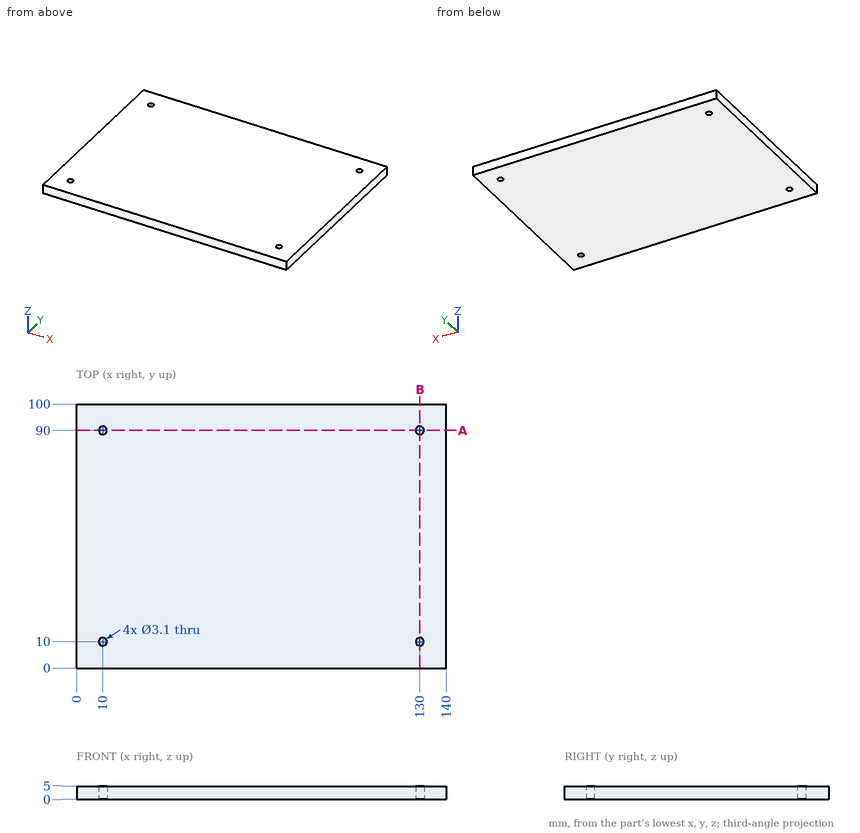
Design review of the part shown in the three views and the two pictorial views. Dimensions are in mm from the part's minimum x, y and z. Give positions to 0.01 mm unless a question says otherwise; leave off trailing zeros. Write each loop counter-clockwise with the first axis right and the second up, starting at its lowest first coordinate (ties: lowest second). Pieces come first, ordered by that corner, then holes.
Item 1: Take a section at A-A (y = 90). Give the boundary of the cut face in (x, z).
Item 2: Wall thickness on probe 1 along X at (y, z) = (90, 3.1); probe 2 along Y at (x, z) = (10, 1.4); probe 3 along X at (y, z) = (91, 3.9): over which ranges is each line inside the solid? List them lowest first.
Item 3: Take a section at B-B (x = 130). Give the boundary of the cut face in (y, z).
Established:
1. outline: (0, 0) - (8.45, 0) - (8.45, 5) - (0, 5) - close; (11.55, 0) - (128.45, 0) - (128.45, 5) - (11.55, 5) - close; (131.55, 0) - (140, 0) - (140, 5) - (131.55, 5) - close
2. probe 1: x = 0 to 8.45, 11.55 to 128.45, 131.55 to 140
2. probe 2: y = 0 to 8.45, 11.55 to 88.45, 91.55 to 100
2. probe 3: x = 0 to 8.82, 11.18 to 128.82, 131.18 to 140
3. outline: (0, 0) - (8.45, 0) - (8.45, 5) - (0, 5) - close; (11.55, 0) - (88.45, 0) - (88.45, 5) - (11.55, 5) - close; (91.55, 0) - (100, 0) - (100, 5) - (91.55, 5) - close
